from build123d import *

# Parameters (mm, degrees)
F0_R     = 1.5
F0_R_2   = 3.5
F1_DEPTH = 2
F3_DEPTH = 25


with BuildPart() as f1:
    # F0 (on Top) → F1 (new body)
    with BuildSketch(Plane.XY):
        with BuildLine():
            ThreePointArc((-67.034419, 13.74533), (-68.448505, 12.054094), (-68.997817, 9.919106))
            ThreePointArc((-68.997817, 9.919106), (-68.531663, 8.911115), (-67.5, 8.5))
            Line((-67.5, 8.5), (-53, 8.5))
            ThreePointArc((-53, 8.5), (-46.989592, 6.010408), (-44.5, 0))
            ThreePointArc((-44.5, 0), (-46.989592, -6.010408), (-53, -8.5))
            Line((-53, -8.5), (-67.5, -8.5))
            ThreePointArc((-67.5, -8.5), (-68.531663, -8.911115), (-68.997817, -9.919106))
            ThreePointArc((-68.997817, -9.919106), (-68.448505, -12.054094), (-67.034419, -13.74533))
            ThreePointArc((-67.034419, -13.74533), (-66.819137, -13.93569), (-66.63336, -14.154938))
            ThreePointArc((-66.63336, -14.154938), (-64.466194, -15.754442), (-61.773732, -15.829696))
            ThreePointArc((-61.773732, -15.829696), (-61.260071, -15.754251), (-60.744298, -15.813559))
            ThreePointArc((-60.744298, -15.813559), (-38.15747, -19.649003), (-15.25, -20))
            Line((-15.25, -20), (15.25, -20))
            ThreePointArc((15.25, -20), (48.882685, -16.940884), (82.110948, -10.907783))
            ThreePointArc((82.110948, -10.907783), (84.908628, -9.150879), (86, -6.032766))
            Line((86, -6.032766), (86, 0))
            Line((86, 0), (86, 6.032766))
            ThreePointArc((86, 6.032766), (84.908628, 9.150879), (82.110948, 10.907783))
            ThreePointArc((82.110948, 10.907783), (48.882685, 16.940884), (15.25, 20))
            Line((15.25, 20), (-15.25, 20))
            ThreePointArc((-15.25, 20), (-38.15747, 19.649003), (-60.744298, 15.813559))
            ThreePointArc((-60.744298, 15.813559), (-61.260071, 15.754251), (-61.773732, 15.829696))
            ThreePointArc((-61.773732, 15.829696), (-64.466194, 15.754442), (-66.63336, 14.154938))
            ThreePointArc((-66.63336, 14.154938), (-66.819137, 13.93569), (-67.034419, 13.74533))
        make_face()
        with Locations((-63, -11.5)):
            Circle(F0_R, mode=Mode.SUBTRACT)
        with Locations((-26, -15.25)):
            Circle(F0_R, mode=Mode.SUBTRACT)
        with Locations((32, -15.25)):
            Circle(F0_R, mode=Mode.SUBTRACT)
        with BuildLine():
            Line((42, -12), (44, -12))
            ThreePointArc((44, -12), (45.5, -13.5), (44, -15))
            Line((44, -15), (42, -15))
            ThreePointArc((42, -15), (40.5, -13.5), (42, -12))
        make_face(mode=Mode.SUBTRACT)
        with BuildLine():
            Line((66.739528, -7.875442), (68.739528, -7.522788))
            ThreePointArc((68.739528, -7.522788), (70.477212, -8.739528), (69.260472, -10.477212))
            Line((69.260472, -10.477212), (67.260472, -10.829866))
            ThreePointArc((67.260472, -10.829866), (65.522788, -9.613126), (66.739528, -7.875442))
        make_face(mode=Mode.SUBTRACT)
        with Locations((81, -6)):
            Circle(F0_R, mode=Mode.SUBTRACT)
        with Locations((-63, 11.5)):
            Circle(F0_R, mode=Mode.SUBTRACT)
        with Locations((-26, 15.25)):
            Circle(F0_R, mode=Mode.SUBTRACT)
        with Locations((73.5, 0)):
            Circle(F0_R_2, mode=Mode.SUBTRACT)
        with Locations((81, 6)):
            Circle(F0_R, mode=Mode.SUBTRACT)
        with BuildLine():
            ThreePointArc((66.739528, 7.875442), (65.522788, 9.613126), (67.260472, 10.829866))
            Line((67.260472, 10.829866), (69.260472, 10.477212))
            ThreePointArc((69.260472, 10.477212), (70.477212, 8.739528), (68.739528, 7.522788))
            Line((68.739528, 7.522788), (66.739528, 7.875442))
        make_face(mode=Mode.SUBTRACT)
        with BuildLine():
            ThreePointArc((42, 12), (40.5, 13.5), (42, 15))
            Line((42, 15), (44, 15))
            ThreePointArc((44, 15), (45.5, 13.5), (44, 12))
            Line((44, 12), (42, 12))
        make_face(mode=Mode.SUBTRACT)
        with Locations((32, 15.25)):
            Circle(F0_R, mode=Mode.SUBTRACT)
    extrude(amount=F1_DEPTH)

    # F2 (on face) → F3 (cut)
    with BuildSketch(Plane.XY.offset(2)):
        with BuildLine():
            Line((-32.997817, 15), (-34.997817, 15))
            ThreePointArc((-34.997817, 15), (-35.497817, 15.5), (-35.997817, 15))
            Line((-35.997817, 15), (-35.997817, 14))
            ThreePointArc((-35.997817, 14), (-35.497817, 13.5), (-34.997817, 14))
            Line((-34.997817, 14), (-32.997817, 14))
            ThreePointArc((-32.997817, 14), (-32.497817, 13.5), (-31.997817, 14))
            Line((-31.997817, 14), (-31.997817, 15))
            ThreePointArc((-31.997817, 15), (-32.497817, 15.5), (-32.997817, 15))
        make_face()
        with BuildLine():
            Line((-35.997817, -14), (-35.997817, -15))
            ThreePointArc((-35.997817, -15), (-35.497817, -15.5), (-34.997817, -15))
            Line((-34.997817, -15), (-32.997817, -15))
            ThreePointArc((-32.997817, -15), (-32.497817, -15.5), (-31.997817, -15))
            Line((-31.997817, -15), (-31.997817, -14))
            ThreePointArc((-31.997817, -14), (-32.497817, -13.5), (-32.997817, -14))
            Line((-32.997817, -14), (-34.997817, -14))
            ThreePointArc((-34.997817, -14), (-35.497817, -13.5), (-35.997817, -14))
        make_face()
    extrude(amount=-F3_DEPTH, mode=Mode.SUBTRACT)


solid = f1.part
Work out the finished part from the listing and answer in its coordinate system (mm). Give positions to 0.01 mm unless a question says otherwise; leave off trailing zeros. Loops run counter-clockwise (first coordinate to the right, second up) from the corner with the lowest first, then second, coordinate; pieces in that order, holes last. Notation, with made-up numbers: (48.5, -18) -> (53.5, -18) arc R21 ccw to (53.5, -13) -> close; hole circle Ø5 at (-27, 58). An arc over 180 degrees is marked (long way). Use a Markdown table: item, result. Add a question column.
1. Find the intervals of material crossed by probe 1 along Y at (x, z) = (-26, 0.8); probe 2 along Y at (x, z) = (42, 0.65); probe 3 along X at (y, z) = (1, 1.7), in increasing order.
2. Determine the mould class of faces 1 (the cylindrical face through (84.94, 9.11, 0.99)), 2 (the cylindrical face through (-61.57, 11.95, 0.99)), 3 (the flat face through (7, 0, 2)) for opening direction X: released by +X, released by -X, zero draft, split by the parting line, or undercut.
3. Section C-C on z = 1.2 is taken. State how many separate pieces and enclosed holes the cut face has, and give its area (3 significant figures).
4. Flat-ended cylindrical pins translate along their axes: pin 1 Ø1 at (x, z) = (43, 1) entering from -Y; pin 2 Ø0.5 at (y, z) = (-14.5, 1.5) entering from -X; pin 3 Ø1 at (x, z) = (53.5, 0.5) entering from +Y. Find the tip coordinate at first contact, or state that the pin passes through.
5. Section B-B on x = -51 is taken. Determine the outline of the cut face in (y, z), and give its area (3 significant figures).
6. Section A-A on x = 32 is taken. Determine the outline of the cut face in (y, z).
7. Section D-D on x = -26 is taken. Determine the outline of the cut face in (y, z).
Results below:
| question | item | result |
|---|---|---|
| 1 | probe 1 | y = -20.27 to -16.75, -13.75 to 13.75, 16.75 to 20.27 |
| 1 | probe 2 | y = -17.81 to -15, -12 to 12, 15 to 17.81 |
| 1 | probe 3 | x = -44.56 to 70.15, 76.85 to 86 |
| 2 | face 1 | released by +X |
| 2 | face 2 | undercut |
| 2 | face 3 | zero draft |
| 3 | separate pieces | 1 |
| 3 | enclosed holes | 15 |
| 3 | area | 4,930 mm^2 |
| 4 | pin 1 | stops at y = -17.75 |
| 4 | pin 2 | stops at x = -66.56 |
| 4 | pin 3 | stops at y = 16.36 |
| 5 | outline | (-17.9, 0) -> (-8.26, 0) -> (-8.26, 2) -> (-17.9, 2) -> close; (8.26, 0) -> (17.9, 0) -> (17.9, 2) -> (8.26, 2) -> close |
| 5 | area | 38.6 mm^2 |
| 6 | outline | (-18.85, 0) -> (-16.75, 0) -> (-16.75, 2) -> (-18.85, 2) -> close; (-13.75, 0) -> (13.75, 0) -> (13.75, 2) -> (-13.75, 2) -> close; (16.75, 0) -> (18.85, 0) -> (18.85, 2) -> (16.75, 2) -> close |
| 7 | outline | (-20.27, 0) -> (-16.75, 0) -> (-16.75, 2) -> (-20.27, 2) -> close; (-13.75, 0) -> (13.75, 0) -> (13.75, 2) -> (-13.75, 2) -> close; (16.75, 0) -> (20.27, 0) -> (20.27, 2) -> (16.75, 2) -> close |
